Geometry check sheet. Reference: the model listing, model coordinates, mm. A direction names the side the tool comes from. Coordinates: 2 decimals unless noted, no trailing zeros. Order: outer loops, then holes, each group sorted by start corner. A loop starts at its lowest first (then second) coordinate and runs counter-clockwise, first axis right, second up. Notation, with made-up numbers: M -34,-35 L 11,-35 A8 cw 11,-30 Z; hole C 16.25,15 d1. An arc over 180 degrees is marked long. One line per item, written item: value. Start each with the question number.
1) Sectioned sample at A-A, the plane z = -10. Enter the section's corners in (x, y).
2) Sectioned sample at D-D, the plane z = -8. Enter the section's corners in (x, y).
3) Sectioned sample at B-B, the plane x = 21. Enter the section's corners in (y, z).
4) Go/stop test with flat-tipped pins: P1, Ø0.9, axis at x = 20.5, z = -13, coming from the -Y side; P2, Ø6.5, axis at y = 7.5, z = -8.5, coming from the +X side; P3, Ø5, axis at x = 6, z = -8.5, coming from the +Y side. Record where each tip stops, or that it passes through.
5) Access from +Z, -Z, +X, -X, +Y, -Y to the whole of each face (thin tool, end or side, straight path). Record for faces 4 (the flat face through (23, 8, -12)), 5 (the flat face through (7, 7, -3)), 6 (the flat face through (23, 3, -1)).
6) Thickness scan on L1, parallel to Z at x = 5.5, y = 6.5; L2, parallel to Z at x = 23.5, y = 4.25; L3, parallel to Y at x = 7.5, z = -10. Record the ranges inside material, lowest first. Write a range as from..to.
7) Sectioned sample at C-C, the plane y = 6.5. Enter the section's corners in (x, z).
8) Draft check along Z on faces 1 (the flat face through (7, 0, -8)), 2 (the flat face through (12, 8, -6)), 3 (the flat face through (15, 7, 0)). Enter one of: pulls with the +Z half, pulls with the -Z half, needs draft (parallel to the pull), parting line crosses it, or undercut.
```python
from build123d import *

# Parameters (mm, degrees)
SKETCH2_W           = 15
SKETCH2_H           = 15
BOSS_EXTRUDE1_DEPTH = 3
BOSS_EXTRUDE2_DEPTH = 3
SKETCH5_W           = 9
SKETCH5_H           = 10
BOSS_EXTRUDE4_DEPTH = 3
CUT_EXTRUDE1_REACH  = 26.88
SKETCH6_R           = 2.5


with BuildPart() as part:
    # Sketch2 → Boss-Extrude1 (new body)
    with BuildSketch(Plane(origin=(0, 0, 0), x_dir=(1, 0, 0), z_dir=(0, 1, 0))):
        with Locations((7.5, 7.5)):
            Rectangle(SKETCH2_W, SKETCH2_H)
    extrude(amount=BOSS_EXTRUDE1_DEPTH)

    # Sketch3 → Boss-Extrude2 (add)
    with BuildSketch(Plane.XY):
        Polygon((0, 3), (10, 13), (30, 13), (30, 3), align=None)
    boss_extrude2 = extrude(amount=-BOSS_EXTRUDE2_DEPTH)

    # Mirror1: Boss-Extrude2 across plane
    add(boss_extrude2.mirror(Plane.XY.offset(-7.5)))

    # Sketch5 → Boss-Extrude4 (add)
    with BuildSketch(Plane(origin=(15, 0, 0), x_dir=(0, 0, -1), z_dir=(1, 0, 0))):
        with Locations((7.5, 8)):
            Rectangle(SKETCH5_W, SKETCH5_H)
    extrude(amount=-BOSS_EXTRUDE4_DEPTH)

    # Sketch6 → Cut-Extrude1 (cut, up to next)
    with BuildSketch(Plane(origin=(15, 0, 0), x_dir=(0, 0, -1), z_dir=(1, 0, 0)), mode=Mode.PRIVATE) as cut_extrude1_sk1:
        with Locations(Location((10, 6.5, 0), (0, 0, 323.130102354))):
            Circle(SKETCH6_R)
    cut_extrude1_tool1 = extrude(cut_extrude1_sk1.sketch, amount=-CUT_EXTRUDE1_REACH, mode=Mode.PRIVATE) & part.part
    add(cut_extrude1_tool1.solids().sort_by_distance((15, 6.5, -10))[0], mode=Mode.SUBTRACT)


solid = part.part
```
Final values:
1. outline: M 0,0 L 15,0 L 15,4 L 12,4 L 12,3 L 0,3 Z; M 12,9 L 15,9 L 15,13 L 12,13 Z
2. outline: M 0,0 L 15,0 L 15,5 L 12,5 L 12,3 L 0,3 Z; M 12,8 L 15,8 L 15,13 L 12,13 Z
3. outline: M 3,-15 L 13,-15 L 13,-12 L 3,-12 Z; M 3,-3 L 13,-3 L 13,0 L 3,0 Z
4. P1: stops at y = 3
4. P2: stops at x = 15
4. P3: stops at y = 3
5. face 4: +X, +Y, -Y
5. face 5: -X, +Y
5. face 6: +Z, -Z, +X, -Y
6. L1: z = -15..-12.5, -3..0
6. L2: z = -15..-12, -3..0
6. L3: y = 0..3
7. outline: M 3.5,-15 L 30,-15 L 30,-12 L 15,-12 L 15,-12.5 L 3.5,-12.5 Z; M 3.5,-3 L 12,-3 L 12,-7.5 L 15,-7.5 L 15,-3 L 30,-3 L 30,0 L 3.5,0 Z
8. face 1: needs draft
8. face 2: undercut
8. face 3: pulls with the +Z half
